Autodesk Inventor part; units mm, degrees
ref_plane "YZ Plane" through (0, 0, 0) normal (1, 0, 0) x (0, 1, 0)
ref_plane "XZ Plane" through (0, 0, 0) normal (0, 1, 0) x (-1, 0, 0)
ref_plane "XY Plane" through (0, 0, 0) normal (0, 0, 1) x (1, 0, 0)
sketch "Sketch12" plane through (0, 0, 0) normal (0, 0, 1) x (1, 0, 0)
  line L0 (-12.5, 15) -> (12.5, 15)
  line L1 (12.5, 15) -> (12.5, -15)
  line L2 (12.5, -15) -> (-12.5, -15)
  line L3 (-12.5, -15) -> (-12.5, 15)
  line L4 (-12.5, 15) -> (12.5, -15) construction
  line L5 (12.5, 15) -> (-12.5, -15) construction
  point P0 (0, 0)
  dimension "d48" = 25
  dimension "d49" = 30
extrude "Extrusion12" add sketch "Sketch12" along normal blind 3
sketch "Sketch15" plane through (0, 0, 0) normal (0, 0, -1) x (-1, 0, 0)
  line L0 (12.5, -15) -> (-12.5, -15) construction
  line L1 (12.5, 15) -> (12.5, -15) construction
  line L2 (-12.5, 15) -> (12.5, 15) construction
  line L3 (-12.5, -15) -> (-12.5, 15) construction
  line L4 (12.5, 0) -> (-12.5, 0) construction
  line L5 (5, 15) -> (-5, 15)
  line L6 (-5, 15) -> (-5, 75)
  line L7 (-5, 75) -> (5, 75)
  line L8 (5, 75) -> (5, 15)
  line L9 (5, -15) -> (-5, -15)
  line L10 (-5, -15) -> (-5, -75)
  line L11 (-5, -75) -> (5, -75)
  line L12 (5, -75) -> (5, -15)
  point P0 (0, 0)
  point P1 (0, 15)
  point P2 (0, 0)
  dimension "d74" = 10
  dimension "d75" = 60
extrude "Extrusion15" add sketch "Sketch15" against normal up to surface (3 mm away)
fillet "Fillet1" radius 4 4 edges at (5, 75, 1.5) (-5, 75, 1.5) (-5, -75, 1.5) (5, -75, 1.5)
sketch "Sketch17" plane through (0, 0, 3) normal (0, 0, 1) x (1, 0, 0)
  line L0 (5.75, 5.75) -> (-5.75, 5.75) construction
  line L1 (-5.75, 5.75) -> (-5.75, -5.75) construction
  line L2 (-5.75, -5.75) -> (5.75, -5.75) construction
  line L3 (5.75, -5.75) -> (5.75, 5.75) construction
  line L4 (5.75, 5.75) -> (-5.75, -5.75) construction
  line L5 (-5.75, 5.75) -> (5.75, -5.75) construction
  line L6 (5.75, 5.75) -> (2.25, 5.75)
  line L7 (2.25, 5.75) -> (2.25, -5.75)
  line L8 (2.25, -5.75) -> (5.75, -5.75)
  line L9 (5.75, -5.75) -> (5.75, 5.75)
  line L10 (-5.75, -5.75) -> (-2.25, -5.75)
  line L11 (-2.25, -5.75) -> (-2.25, 5.75)
  line L12 (-2.25, 5.75) -> (-5.75, 5.75)
  line L13 (-5.75, 5.75) -> (-5.75, -5.75)
  point P0 (0, 0)
  dimension "d84" = 11.5
  dimension "d85" = 11.5
  dimension "d86" = 3.5
  dimension "d87" = 3.5
extrude "Extrusion17" add sketch "Sketch17" along normal blind 12
sketch "Sketch18" plane through (-5.75, -5.75, 3) normal (0, -1, 0) x (1, 0, 0)
  line L0 (3.5, 0) -> (0, 0) construction
  line L1 (3.5, 0) -> (3.5, 12) construction
  line L2 (0, 12) -> (3.5, 12) construction
  line L3 (0, 0) -> (0, 12) construction
  line L4 (11.5, 0) -> (8, 0) construction
  line L5 (11.5, 0) -> (11.5, 12) construction
  line L6 (8, 12) -> (11.5, 12) construction
  line L7 (8, 0) -> (8, 12) construction
  line L8 (0, 10) -> (11.5, 10)
  line L9 (11.5, 10) -> (11.5, 7)
  line L10 (11.5, 7) -> (0, 7)
  line L11 (0, 7) -> (0, 10)
  point P0 (5.75, -3)
  dimension "d90" = 2
  dimension "d91" = 3
extrude "Extrusion18" cut sketch "Sketch18" against normal blind 5
properties part number "base"
Here's how the part is built. I have some questions about the finished solid (model axes, mm). A direction names the side the tool comes from. Round coordinates to 2 decimals unless told otherwise and drop trailing zeros. Order: outer loops, then holes, each group sorted by start corner. A loop starts at its lowest first (then second) coordinate and runs counter-clockwise, first axis right, second up. Notation, with made-up numbers: M 30.25,77.25 L 87.25,77.25 A23 ccw 87.25,86.25 Z; hole C 69,44 d10. An arc over 180 degrees is marked long. Return JSON: item names as keys, results as strings. Group by question number.
1. Please list where these lines run through material, in increasing order: probe 1 along Z at (x, y) = (-3, -61.5); probe 2 along Y at (x, z) = (8.5, 2.75); probe 3 along Y at (x, z) = (2.5, 13.25).
2. If we section it at C-C on x = -3.5: List the corners of the cut face in (y, z) for me, then the cut area to 3 significant figures.
3. If we section it at D-D on y = -10: List the corners of the cut face in (x, z) for me, then the cut area to 3 significant figures.
4. I'm going to push flat-ended pins straight in: pin 1 Ø4 at (x, z) = (-3, 7.5) entering from -Y; pin 2 Ø9 at (y, z) = (2, 11) entering from +X; pin 3 Ø6 at (x, y) = (4, 34) entering from +Z; pin 4 Ø3 at (x, y) = (-4, -2.5) entering from -Z. Where does each tip first touch, or does it pass through?
5. If we mould it in two halves opening along X, with no side actions, what happens to faces 1 (the face through (-9, -15, 1)), 2 (the face through (-5.75, 0, 9)), 3 (the face through (2.25, 0, 9)), 4 (the face through (3.859, 73.797, 1.521))? For each: pulls with the +X half, pulls with the -X half, needs draft (parallel to the pull), parting line crosses it, or undercut.
6. If we section it at B-B on z = 1.75: List the corners of the cut face in (x, y) for me.
7. If we section it at A-A on z = 11.25: List the corners of the cut face in (x, y) for me, then the cut area to 3 significant figures.
8. On a 3-axis mill with a long thin cutter (end or side, diameter ignored), from which of +Z, -Z, +X, -X, +Y, -Y can I reach the whole of each face in a straight line? I mean faces 5 (the face through (-4, -5.75, 6)), 6 (the face through (-2.25, 0, 9)), 7 (the face through (5, -43, 1)), 8 (the face through (4, -0.75, 12)), 9 (the face through (-9, 15, 1)). Say none if no direction works.
Reply:
{
 "1": {"probe 1": "0 to 3", "probe 2": "-15 to 15", "probe 3": "-5.75 to 5.75"},
 "2": {"outline": "M -74.12,0 L 74.12,0 L 74.12,3 L 5.75,3 L 5.75,15 L -5.75,15 L -5.75,13 L -0.75,13 L -0.75,10 L -5.75,10 L -5.75,3 L -74.12,3 Z", "area": "568 mm^2"},
 "3": {"outline": "M -12.5,0 L 12.5,0 L 12.5,3 L -12.5,3 Z", "area": "75.0 mm^2"},
 "4": {"pin 1": "y = -5.75", "pin 2": "x = 5.75", "pin 3": "z = 3", "pin 4": "z = 0"},
 "5": {"face 1": "needs draft", "face 2": "pulls with the -X half", "face 3": "undercut", "face 4": "pulls with the +X half"},
 "6": {"outline": "M -12.5,-15 L -5,-15 L -5,-71 A4 ccw -1,-75 L 1,-75 A4 ccw 5,-71 L 5,-15 L 12.5,-15 L 12.5,15 L 5,15 L 5,71 A4 ccw 1,75 L -1,75 A4 ccw -5,71 L -5,15 L -12.5,15 Z"},
 "7": {"outline": "M -5.75,-0.75 L -2.25,-0.75 L -2.25,5.75 L -5.75,5.75 Z; M 2.25,-0.75 L 5.75,-0.75 L 5.75,5.75 L 2.25,5.75 Z", "area": "45.5 mm^2"},
 "8": {"face 5": "+Z, +X, -X, -Y", "face 6": "+Z, +Y, -Y", "face 7": "+Z, -Z, +X, -Y", "face 8": "+X, -X, -Y", "face 9": "+Z, -Z, -X, +Y"}
}
